Input: part model. Units: mm. Frame: model coordinates. Coordinates: 2 decimals unless noted, no trailing zeros. Loops run counter-clockwise (first coordinate to the right, second up) from the corner with the lowest first, then second, coordinate; pieces in that order, holes last.
(1) Contact query for flat-ended pins moving along their axis: P1, Ø2.5, axis at x = 22, z = 1.5, coming from the +Y side; P2, Ø4.5, axis at x = -17.85, y = 19.9, coming from the -Z side; P3, Ø2, axis at x = 7, y = 20.5, coming from the -Z side; P4, Ø3.5, axis at y = -2, z = 1, coming from the -X side. Output: stop coordinate, or through.
(2) Line query: L1, parallel to Z at x = -19.5, y = 14.5; L2, parallel to Y at x = 33, z = 2.25; L3, parallel to X at y = -6, z = 0.75. Output: solid intervals per line, ascending.
(3) Section B-B, the plane y = -20.5. Return loops of the section in (x, z), then the cut area to 3 significant figures.
(4) Section D-D, the plane z = -5. Return loops of the section in (x, y), then the cut area to 3 significant figures.
(5) Section C-C, the plane z = 1.75. Return loops of the section in (x, y), then the cut area to 3 significant figures.
(6) Section A-A, the plane x = -36. Return loops of the section in (y, z).
```python
from build123d import *

# Parameters (mm, degrees)
SKETCH_2_R       = 2.5
SKETCH_2_R_2     = 4
SKETCH_2_R_3     = 2
EXTRUDE_11_DEPTH = 3
SKETCH_2_16_R    = 4
SKETCH_2_16_R_2  = 2
EXTRUDE_12_DEPTH = 0.5
SKETCH_2_17_R    = 2
EXTRUDE_13_DEPTH = 12.5
FILLET_1_R       = 0.3


with BuildPart() as part:
    # Sketch 2 → Extrude 11 (new body)
    # profile 1 of 7: a face of its own
    with BuildSketch(Plane.XY):
        Polygon((-41.985987982, 15.322651266), (-41.985987982, 21.467672234), (-25.900833035, 21.467672234), (-21.525354797, 25.843150472), (-14.576398582, 25.843150472), (-9.421808725, 23.655411353), (34.384238258, 23.655411353), (40.290588771, 21.148605879), (40.290588771, -26.048068749), (-41.985987982, -26.048068749), (-41.985987982, -12.123358681), (-33.943410509, -12.123358681), (-33.943410509, 11.301362529), (-37.964699246, 11.301362529), align=None)
        with Locations((9.574246485, 7.73050044)):
            Circle(SKETCH_2_R, mode=Mode.SUBTRACT)
        with Locations((-8.153758739, -18.910029411)):
            Circle(SKETCH_2_R, mode=Mode.SUBTRACT)
        with Locations((24.574246485, 17.73050044)):
            Circle(SKETCH_2_R_2, mode=Mode.SUBTRACT)
        with Locations((-29.162107176, 7.874269984)):
            Circle(SKETCH_2_R_2, mode=Mode.SUBTRACT)
        with Locations((-17.847699606, 19.897540861)):
            Circle(SKETCH_2_R, mode=Mode.SUBTRACT)
        with BuildLine():
            Line((24.695702599, -6.26949956), (30.574246485, -6.26949956))
            ThreePointArc((30.574246485, -6.26949956), (31.281353266, -5.976606341), (31.574246485, -5.26949956))
            Line((31.574246485, -5.26949956), (31.574246485, 0.609044326))
            ThreePointArc((31.574246485, 0.609044326), (31.228514311, 1.365307251), (30.430379263, 1.598641326))
            ThreePointArc((30.430379263, 1.598641326), (25.952143977, -0.647397052), (23.706105599, -5.125632338))
            ThreePointArc((23.706105599, -5.125632338), (23.939439675, -5.923767386), (24.695702599, -6.26949956))
        make_face(mode=Mode.SUBTRACT)
    # profile 2 of 7: a face of its own
    with BuildSketch(Plane.XY):
        with Locations((-29.162107176, 7.874269984)):
            Circle(SKETCH_2_R_2)
        with Locations((-29.162107176, 7.874269984)):
            Circle(SKETCH_2_R_3, mode=Mode.SUBTRACT)
    # profile 3 of 7: a face of its own
    with BuildSketch(Plane.XY):
        with Locations((-29.162107176, 7.874269984)):
            Circle(SKETCH_2_R_3)
    # profile 4 of 7: a face of its own
    with BuildSketch(Plane.XY):
        with Locations((24.574246485, 17.73050044)):
            Circle(SKETCH_2_R_2)
        with Locations((24.574246485, 17.73050044)):
            Circle(SKETCH_2_R_3, mode=Mode.SUBTRACT)
    # profile 5 of 7: a face of its own
    with BuildSketch(Plane.XY):
        with Locations((24.574246485, 17.73050044)):
            Circle(SKETCH_2_R_3)
    # profile 6 of 7: a face of its own
    with BuildSketch(Plane.XY):
        with BuildLine():
            ThreePointArc((24.695702599, -6.26949956), (23.939439675, -5.923767386), (23.706105599, -5.125632338))
            ThreePointArc((23.706105599, -5.125632338), (25.952143977, -0.647397052), (30.430379263, 1.598641326))
            ThreePointArc((30.430379263, 1.598641326), (31.228514311, 1.365307251), (31.574246485, 0.609044326))
            Line((31.574246485, 0.609044326), (31.574246485, -5.26949956))
            ThreePointArc((31.574246485, -5.26949956), (31.281353266, -5.976606341), (30.574246485, -6.26949956))
            Line((30.574246485, -6.26949956), (24.695702599, -6.26949956))
        make_face()
        with Locations((28.616748621, -3.312001696)):
            Circle(SKETCH_2_R_3, mode=Mode.SUBTRACT)
    # profile 7 of 7: a face of its own
    with BuildSketch(Plane.XY):
        with Locations((28.616748621, -3.312001696)):
            Circle(SKETCH_2_R_3)
    extrude(amount=EXTRUDE_11_DEPTH)

    # Sketch 2_16 → Extrude 12 (add)
    # profile 1 of 3: a face of its own
    with BuildSketch(Plane.XY):
        with Locations((-29.162107176, 7.874269984)):
            Circle(SKETCH_2_16_R)
        with Locations((-29.162107176, 7.874269984)):
            Circle(SKETCH_2_16_R_2, mode=Mode.SUBTRACT)
    # profile 2 of 3: a face of its own
    with BuildSketch(Plane.XY):
        with Locations((24.574246485, 17.73050044)):
            Circle(SKETCH_2_16_R)
        with Locations((24.574246485, 17.73050044)):
            Circle(SKETCH_2_16_R_2, mode=Mode.SUBTRACT)
    # profile 3 of 3: a face of its own
    with BuildSketch(Plane.XY):
        with BuildLine():
            ThreePointArc((24.695702599, -6.26949956), (23.939439675, -5.923767386), (23.706105599, -5.125632338))
            ThreePointArc((23.706105599, -5.125632338), (25.952143977, -0.647397052), (30.430379263, 1.598641326))
            ThreePointArc((30.430379263, 1.598641326), (31.228514311, 1.365307251), (31.574246485, 0.609044326))
            Line((31.574246485, 0.609044326), (31.574246485, -5.26949956))
            ThreePointArc((31.574246485, -5.26949956), (31.281353266, -5.976606341), (30.574246485, -6.26949956))
            Line((30.574246485, -6.26949956), (24.695702599, -6.26949956))
        make_face()
        with Locations((28.616748621, -3.312001696)):
            Circle(SKETCH_2_16_R_2, mode=Mode.SUBTRACT)
    extrude(amount=-EXTRUDE_12_DEPTH)

    # Sketch 2_17 → Extrude 13 (add)
    with BuildSketch(Plane.XY):
        with Locations((28.616748621, -3.312001696)):
            Circle(SKETCH_2_17_R)
        with Locations((24.574246485, 17.73050044)):
            Circle(SKETCH_2_17_R)
        with Locations((-29.162107176, 7.874269984)):
            Circle(SKETCH_2_17_R)
    extrude(amount=-EXTRUDE_13_DEPTH)

    # Fillet 1
    fillet_1_edges = [part.edges().sort_by_distance(p)[0] for p in [
        (26.616748621, -3.312001696, -12.5),
        (22.574246485, 17.73050044, -12.5),
        (-31.162107176, 7.874269984, -12.5),
    ]]
    fillet(fillet_1_edges, radius=FILLET_1_R)


solid = part.part
```
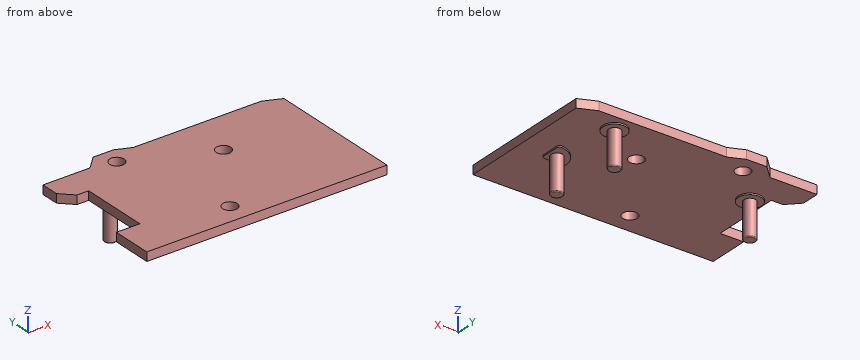
Report:
1. P1: stops at y = 23.66
1. P2: passes through
1. P3: stops at z = 0
1. P4: stops at x = -33.94
2. L1: z = 0 to 3
2. L2: y = -26.05 to 23.66
2. L3: x = -33.94 to 40.29
3. outline: (-41.99, 0) - (-10.08, 0) - (-10.08, 3) - (-41.99, 3) - close; (-6.22, 0) - (40.29, 0) - (40.29, 3) - (-6.22, 3) - close
3. area: 235 mm2
4. outline: circle Ø4 at (-29.16, 7.87); circle Ø4 at (24.57, 17.73); circle Ø4 at (28.62, -3.31)
4. area: 37.7 mm2
5. outline: (-41.99, -26.05) - (40.29, -26.05) - (40.29, 21.15) - (34.38, 23.66) - (-9.42, 23.66) - (-14.58, 25.84) - (-21.53, 25.84) - (-25.9, 21.47) - (-41.99, 21.47) - (-41.99, 15.32) - (-37.96, 11.3) - (-33.94, 11.3) - (-33.94, -12.12) - (-41.99, -12.12) - close; hole circle Ø5 at (-17.85, 19.9); hole circle Ø5 at (-8.15, -18.91); hole circle Ø5 at (9.57, 7.73)
5. area: 3,810 mm2
6. outline: (-26.05, 0) - (-12.12, 0) - (-12.12, 3) - (-26.05, 3) - close; (11.3, 0) - (21.47, 0) - (21.47, 3) - (11.3, 3) - close
